The figure shows three views and two pictorial views of one solid part (mm, origin at its lowest corner). Answer the questions. A direction names the side the tool comes from. Give positions to 0.01 mm unless a question says otherwise; leave off trailing zeros. Order: outer loops, then holes, each group sorted by start corner. A loop starts at its lowest first (then second) coordinate and runs counter-clockwise, first axis right, second up. Notation, with made-up numbers: (0.25, 0) -> (32.25, 0) arc R27 cw to (32.25, 19) -> close; hole circle Ø5 at (81.5, -16). An arc over 180 degrees is marked (long way). Use one line per item in the form item = value.
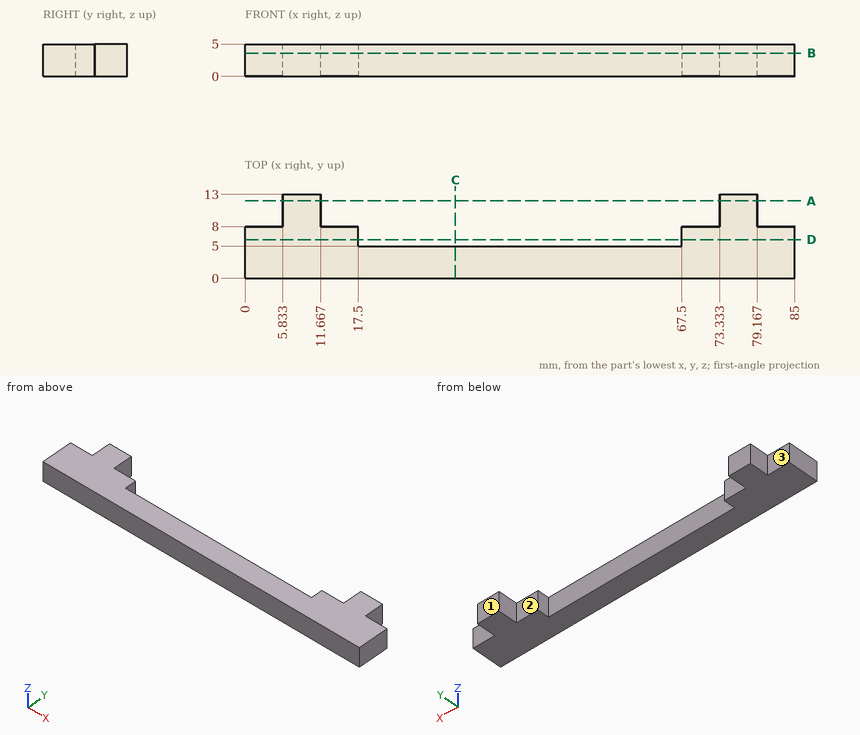
Item 1: The part is cut by section D-D on y = 6. Give the vertices of the cut face in (x, z).
Checks:
outline = (0, 0) -> (17.5, 0) -> (17.5, 5) -> (0, 5) -> close; (67.5, 0) -> (85, 0) -> (85, 5) -> (67.5, 5) -> close
Item 2: The part is cut by section A-A on y = 12. Give the vertices of the cut face in (x, z).
Checks:
outline = (5.83, 0) -> (11.67, 0) -> (11.67, 5) -> (5.83, 5) -> close; (73.33, 0) -> (79.17, 0) -> (79.17, 5) -> (73.33, 5) -> close
Item 3: The part is cut by section B-B on z = 3.6. Give the vertices of the cut face in (x, y), and give its area (3 significant figures).
Checks:
outline = (0, 0) -> (85, 0) -> (85, 8) -> (79.17, 8) -> (79.17, 13) -> (73.33, 13) -> (73.33, 8) -> (67.5, 8) -> (67.5, 5) -> (17.5, 5) -> (17.5, 8) -> (11.67, 8) -> (11.67, 13) -> (5.83, 13) -> (5.83, 8) -> (0, 8) -> close
area = 588 mm²
Item 4: Given pin 1 Ø2 at (y, z) = (11.5, 3.5) entering from +X; pin 2 Ø1.5 at (x, z) = (72, 2) entering from +Y; pin 3 Ø1.5 at (y, z) = (10, 2.5) entering from -X, each flat-ended and moving along its own axis, determine where each tip first touches the part or whether it passes through.
Checks:
pin_1 = 79.17
pin_2 = 8
pin_3 = 5.83
Item 5: Which of the six approach directions +Z, -Z, +X, -X, +Y, -Y give full straight-line access (tool end or side, diameter ignored) to the marked faces 1, 2 and 3?
Checks:
face_1 = +Z, -Z, +X, -X, +Y
face_2 = +Z, -Z, +Y
face_3 = +Z, -Z, -X, +Y
Item 6: The part is cut by section C-C on x = 32.5. Give the vertices of the cut face in (y, z), and give its area (3 significant figures).
Checks:
outline = (0, 0) -> (5, 0) -> (5, 5) -> (0, 5) -> close
area = 25.0 mm²
Item 7: Straight lines are drawn through the part: L1, parallel to X at y = 10.25, z = 0.75; L2, parallel to X at y = 6.5, z = 4.85; L3, parallel to Y at x = 52, z = 3.2. For each, find the intervals that lie inside material, in ascending order. Write a range as from..to.
Checks:
L1 = 5.83..11.67, 73.33..79.17
L2 = 0..17.5, 67.5..85
L3 = 0..5
